For this review, take the finished solid that the model builds, in its own axes (mm). A direction names the side the tool comes from. Coordinates: 2 decimals unless noted, no trailing zeros. Loops run counter-clockwise (first coordinate to the right, second up) from the corner with the lowest first, then second, coordinate; pieces in that order, holes last. Notation, with made-up numbers: M 40,-22.5 L 69,-22.5 A12 ccw 69,-6.5 Z; hole C 3.25,45.5 d7. An arc over 180 degrees is marked long. Put each result on its own line as item: value.
```python
from build123d import *

# Parameters (mm, degrees)
F0_R     = 26.5
F1_DEPTH = 35
F0_R_2   = 31.673016
F2_DEPTH = 5
F3_D     = 8.5


with BuildPart() as f1:
    # F0 (on Top) → F1 (new body)
    with BuildSketch(Plane.XY):
        Circle(F0_R)
    extrude(amount=F1_DEPTH)

    # F0 (on Top) → F2 (join)
    with BuildSketch(Plane.XY):
        Circle(F0_R_2)
        Circle(F0_R, mode=Mode.SUBTRACT)
    extrude(amount=F2_DEPTH)

    # F3 (through all)
    with Locations(Plane(origin=(0, 0, 0), x_dir=(1, 0, 0), z_dir=(0, 0, -1))):
        with Locations((0, 0)):
            Hole(F3_D / 2)


solid = f1.part
```
(1) Wall thickness on line 1 along Y through (x, z) = (0, 22); line 2 along Z through (x, y) = (24, -20.5); line 3 along Y through (x, z) = (1, 11.5): over which ranges is each line inside the solid? List them lowest first. Write a range as [from, to].
Determined:
line 1: y = [-26.5, -4.25], [4.25, 26.5]
line 2: z = [0, 5]
line 3: y = [-26.48, -4.13], [4.13, 26.48]
(2) Draft analysis for pull direction Y (two halves, no side actions). For faces 3 (the flat face through (6, 0, 35)), 4 (the cylindrical face through (-2.285, -3.584, 17.745)), 5 (the cylindrical face through (14.246, 22.345, 19.79)), state which applies: +Y half, -Y half, draft (parallel to the pull), parting line (faces both ways), or undercut.
Determined:
face 3: draft
face 4: undercut
face 5: parting line
(3) Add section C-C (z = 11.5). Write out the cut boundary in (x, y).
Determined:
outline: C 0,0 d53; hole C 0,0 d8.5
(4) Tool access review of faces 1 (the flat face through (7, 0, 0)), 2 (the flat face through (-7, -26, 5)): name each direction out of +Z, -Z, +X, -X, +Y, -Y from which nothing blocks a thin tool from reaching the whole face with its end or side.
Determined:
face 1: -Z, +X, -X, +Y, -Y
face 2: +Z
(5) Add section A-A (y = 0). Write out the cut boundary in (x, z).
Determined:
outline: M -31.67,0 L -4.25,0 L -4.25,35 L -26.5,35 L -26.5,5 L -31.67,5 Z; M 4.25,0 L 31.67,0 L 31.67,5 L 26.5,5 L 26.5,35 L 4.25,35 Z
(6) For pin 1 (6 mm diameter, centred on y = 11.5, z = 25.5, fed in from +X); pin 2 (2 mm diameter, centred on x = 23.5, y = -21, fed in from +Z); pin 3 (6 mm diameter, centred on x = 3.5, z = 30, fed in from +Y), all flat-tipped, find the tip position at first contact; note any pin that passes through.
Determined:
pin 1: stops at x = 25.1
pin 2: stops at z = 5
pin 3: stops at y = 26.5
(7) Add section D-D (y = 15.5). Write out the cut boundary in (x, z).
Determined:
outline: M -27.62,0 L 27.62,0 L 27.62,5 L 21.49,5 L 21.49,35 L -21.49,35 L -21.49,5 L -27.62,5 Z
